Can you work these out from the model? Positions are in its coordinate system, mm. A direction names the side the tool comes from. Round coordinates to 2 decimals unless told otherwise and drop trailing zeros. Order: outer loops, then holes, each group sorted by start corner. A loop starts at its lowest first (then second) coordinate and runs counter-clockwise, first axis right, second up. Notation, with made-up numbers: (41.5, 39) -> (100.5, 39) arc R30 cw to (100.5, 67) -> close; hole circle Ø4 at (-34, 25.25). An arc over 180 degrees is marked (long way). Use a Markdown table: item, result. Add a question column.
Q1. I need wall thicknesses on line 1 along X through (y, z) = (11.5, 0); line 2 along Y through (x, z) = (-1.25, -2.5); line 3 along Y through (x, z) = (0.75, -2.5). Which ranges of each line are inside material? Lowest first, please. Write a range as [from, to].
Q2. I'm going to push a flat-ended pin straight in: pin 1 Ø2 at (x, y) = (1, 10) entering from +Z. Where does the tip first touch, or does it pass through?
Q3. For faces 1 (the face through (0, 0, 0)), 2 (the face through (-0.944, 11.536, 0.124)), which set-ups out of +Z, -Z, +X, -X, +Y, -Y let a thin tool reach every point of the face, with its end or its side?
Q4. If we section it at A-A on y = 15.25: List the corners of the cut face in (x, z) for me (1 decimal).
```python
from build123d import *

# Parameters (mm, degrees)
SKETCH1_R           = 3.048
BOSS_EXTRUDE1_DEPTH = 1.27
SKETCH2_R           = 0.9525
SKETCH3_R           = 0.9525
BOSS_EXTRUDE2_DEPTH = 14.732
FILLET1_R           = 2.54


with BuildPart() as part:
    # Sketch1 → Boss-Extrude1 (new body)
    with BuildSketch(Plane(origin=(0, 0, 0), x_dir=(1, 0, 0), z_dir=(0, 1, 0))):
        with Locations(Location((0, 0, 0), (0, 0, 270))):
            Circle(SKETCH1_R)
    extrude(amount=BOSS_EXTRUDE1_DEPTH)

    # Sketch2 → section 0 of loft1
    with BuildSketch(Plane(origin=(0, 3.81, 0), x_dir=(1, 0, 0), z_dir=(0, 1, 0)), mode=Mode.PRIVATE) as loft1_s0:
        Circle(SKETCH2_R)
    # loft up to a face of the part (loft1)
    loft([loft1_s0.sketch, Face(Wire([part.edges().sort_by_distance((2.221896376, 1.27, -2.086499579))[0]]))])

    # Sketch3 → Boss-Extrude2 (add)
    with BuildSketch(Plane(origin=(0, 3.81, 0), x_dir=(1, 0, 0), z_dir=(0, 1, 0))):
        with Locations(Location((0, 0, 0), (0, 0, 90))):
            Circle(SKETCH3_R)
    extrude(amount=BOSS_EXTRUDE2_DEPTH)

    # Fillet1
    fillet1_edges = [part.edges().sort_by_distance(p)[0] for p in [
        (-2.155261469, 1.27, -2.155261469),
        (-0.673519209, 3.81, 0.673519209),
    ]]
    fillet(fillet1_edges, radius=FILLET1_R)


solid = part.part
```
Answer below:
| question | item | result |
|---|---|---|
| 1 | line 1 | [-0.95, 0.95] |
| 1 | line 2 | [0, 1.46] |
| 1 | line 3 | [0, 1.78] |
| 2 | pin 1 | z = 0.95 |
| 3 | face 1 | +Z, -Z, +X, -X, -Y |
| 3 | face 2 | +Y |
| 4 | outline | circle Ø1.9 at (0, 0) |
